Read the model definition and answer for the solid it produces. Units are mm, in the model's axes. A direction names the side the tool comes from. Give positions to 0.01 mm unless a question says otherwise; leave off trailing zeros. Order: outer loops, then holes, each group sorted by start corner. A loop starts at its lowest first (then second) coordinate and runs counter-clockwise, first axis right, second up. Notation, with made-up numbers: (42.25, -22) - (70.25, -22) arc R20 ccw to (70.25, -18) - close; hole circle Ø11 at (84.25, -31). An arc over 180 degrees is marked (long way). One line per item, written item: value. Start each with the question number.
```python
from build123d import *

# Parameters (mm, degrees)
BOSS_EXTRUDE1_DEPTH  = 60
BOSS_EXTRUDE2_DEPTH  = 15
BOSS_EXTRUDE4_DEPTH  = 15
CUT_EXTRUDE3_DEPTH   = 25
CUT_EXTRUDE4_DEPTH   = 25
FILLET2_R            = 5
FILLET3_R            = 5
SKETCH10_W           = 100
SKETCH10_H           = 30
CUT_EXTRUDE8_DEPTH   = 15
SKETCH12_W           = 100
SKETCH12_H           = 30
BOSS_EXTRUDE10_DEPTH = 1


with BuildPart() as part:
    # Sketch1 → Boss-Extrude1 (new body)
    with BuildSketch(Plane.XY):
        Polygon((-74.571428571, -3.428571429), (-74.571428571, 11.571428571), (15.428571429, 11.571428571), (15.428571429, -3.428571429), (20.428571429, -3.428571429), (20.428571429, 26.571428571), (-79.571428571, 26.571428571), (-79.571428571, -3.428571429), align=None)
    extrude(amount=-BOSS_EXTRUDE1_DEPTH)

    # Sketch3 → Boss-Extrude2 (add)
    with BuildSketch(Plane(origin=(0, 0, -60), x_dir=(-1, 0, 0), z_dir=(0, 0, -1))):
        with BuildLine():
            Line((29.571428571, 26.571428571), (79.571428571, 26.571428571))
            ThreePointArc((79.571428571, 26.571428571), (54.571428571, 51.571428571), (29.571428571, 26.571428571))
        make_face()
    extrude(amount=-BOSS_EXTRUDE2_DEPTH)

    # Sketch4 → Boss-Extrude4 (add)
    with BuildSketch(Plane.XY):
        with BuildLine():
            Line((20.428571429, 26.571428571), (-29.571428571, 26.571428571))
            ThreePointArc((-29.571428571, 26.571428571), (-4.571428571, 51.571428571), (20.428571429, 26.571428571))
        make_face()
    extrude(amount=-BOSS_EXTRUDE4_DEPTH)

    # Sketch5 → Cut-Extrude3 (cut)
    with BuildSketch(Plane.XY):
        with BuildLine():
            Line((-27.48668728, 27.787723549), (18.843123445, 27.787723549))
            ThreePointArc((18.843123445, 27.787723549), (-4.321781917, 48.729240211), (-27.48668728, 27.787723549))
        make_face()
    extrude(amount=-CUT_EXTRUDE3_DEPTH, mode=Mode.SUBTRACT)

    # Sketch6 → Cut-Extrude4 (cut)
    with BuildSketch(Plane.XY.offset(-45)):
        with BuildLine():
            Line((-76.657542496, 28.868881688), (-32.592047201, 28.868881688))
            ThreePointArc((-32.592047201, 28.868881688), (-54.624794848, 49.768229308), (-76.657542496, 28.868881688))
        make_face()
    extrude(amount=-CUT_EXTRUDE4_DEPTH, mode=Mode.SUBTRACT)

    # Fillet2
    fillet2_edges = [part.edges().sort_by_distance(p)[0] for p in [
        (-79.571428571, 26.571428571, -22.5),
    ]]
    fillet(fillet2_edges, radius=FILLET2_R)

    # Fillet3
    fillet3_edges = [part.edges().sort_by_distance(p)[0] for p in [
        (20.428571429, 26.571428571, -37.5),
    ]]
    fillet(fillet3_edges, radius=FILLET3_R)

    # Sketch10 → Cut-Extrude8 (cut)
    with BuildSketch(Plane(origin=(0, 26.571428571, 0), x_dir=(1, 0, 0), z_dir=(0, 1, 0))):
        with Locations((-29.571428571, 30)):
            Rectangle(SKETCH10_W, SKETCH10_H)
    extrude(amount=-CUT_EXTRUDE8_DEPTH, mode=Mode.SUBTRACT)

    # Sketch12 → Boss-Extrude10 (add)
    with BuildSketch(Plane(origin=(0, 11.571428571, 0), x_dir=(1, 0, 0), z_dir=(0, 1, 0))):
        with Locations((-29.571428571, 30)):
            Rectangle(SKETCH12_W, SKETCH12_H)
    extrude(amount=BOSS_EXTRUDE10_DEPTH)


solid = part.part
```
1) Find the intervals of material crossed by probe 1 along X at (y, z) = (7, -23); probe 2 along Z at (x, y) = (-33.5, 18); probe 3 along Y at (x, z) = (-20, -49.5), in increasing order. Write a range as from..to.
2) Section A-A on y = 8 is taken. Write down the section's boundary in (x, z).
3) Section C-C on x = -16 is taken. Write down the section's boundary in (y, z), plus the area to 3 significant figures.
4) Section D-D on y = 34 is taken. Write down the section's boundary in (x, z), plus the area to 3 significant figures.
5) For faces 4 (the cylindrical face through (18.925, 25.146, -52.605)), 5 (the flat face through (-29, 24, -15)), 6 (the flat face through (-30, 11.571, -30)), 7 (the flat face through (-5, 27.788, -7)), 8 (the cylindrical face through (-78.068, 25.146, -7.605)), determine the directions among +Z, -Z, +X, -X, +Y, -Y from which every point of the face is accessible in a straight line to the end or side of a thin tool.
6) Section B-B on z = -8.5 is taken. Write down the section's boundary in (x, y).
7) The mould has two halves that part along Y. Classify faces 1 (the flat face through (-77, -3.429, -30)), 2 (the flat face through (-55, 28.869, -52)), 3 (the flat face through (-29, 18, 0)): +Y half, -Y half, draft (parallel to the pull), parting line (faces both ways), or undercut.
8) Each of these flat-tipped pins is pushed along its axis until it touches: pin 1 (4.5 mm diameter, centred on x = 2.5, z = -49.5, fed in from +Y); pin 2 (2 mm diameter, centred on x = -21, y = 41, fed in from -Z); pin 3 (12 mm diameter, centred on x = 10.5, z = -12, fed in from +Y); pin 4 (6 mm diameter, centred on x = -13, y = 10.5, fed in from -Z). Where does it stop, or does it pass through?
Solved:
1. probe 1: x = -79.57..-74.57, 15.43..20.43
1. probe 2: z = -60..-45, -15..0
1. probe 3: y = 11.57..26.57
2. outline: (-79.57, -60) - (-74.57, -60) - (-74.57, 0) - (-79.57, 0) - close; (15.43, -60) - (20.43, -60) - (20.43, 0) - (15.43, 0) - close
3. outline: (11.57, -60) - (26.57, -60) - (26.57, -45) - (12.57, -45) - (12.57, -15) - (27.79, -15) - (27.79, 0) - (11.57, 0) - close; (45.59, -15) - (48.81, -15) - (48.81, 0) - (45.59, 0) - close
3. area: 547 mm2
4. outline: (-78.44, -60) - (-75.77, -60) - (-75.77, -45) - (-78.44, -45) - close; (-33.48, -60) - (-30.7, -60) - (-30.7, -45) - (-33.48, -45) - close; (-28.44, -15) - (-25.98, -15) - (-25.98, 0) - (-28.44, 0) - close; (17.33, -15) - (19.3, -15) - (19.3, 0) - (17.33, 0) - close
4. area: 148 mm2
5. face 4: -Z, +X, +Y
5. face 5: +X, -X, +Y
5. face 6: +Z, -Z, -Y
5. face 7: +Z, -Z
5. face 8: +Z, -X, +Y
6. outline: (-79.57, -3.43) - (-74.57, -3.43) - (-74.57, 11.57) - (15.43, 11.57) - (15.43, -3.43) - (20.43, -3.43) - (20.43, 26.57) arc R25 ccw to (-29.57, 26.57) - (-74.57, 26.57) arc R5 ccw to (-79.57, 21.57) - close; hole (-27.49, 27.79) - (18.84, 27.79) arc R23.28 ccw to start
7. face 1: -Y half
7. face 2: undercut
7. face 3: draft
8. pin 1: stops at y = 26.57
8. pin 2: stops at z = -15
8. pin 3: stops at y = 49.87
8. pin 4: stops at z = -60
